Answer from the drawing. Dimensions are ordinates in mm from the lowest x, y and z of the part. A direction names the side the tool comes from. Coordinates: 2 decimals unless noted, no trailing zeros. Order: outer loops, then holes, each group sorted by start corner. A loop starts at its lowest first (then second) coordinate and runs counter-clockwise, first axis right, second up. Notation, with made-up numbers: (18.25, -28.75) -> (38.25, -28.75) arc R10 cw to (38.25, -11.75) -> close; hole circle Ø10 at (48, 78). An arc over 180 degrees is marked (long way). Answer in a Markdown table with one row per item.
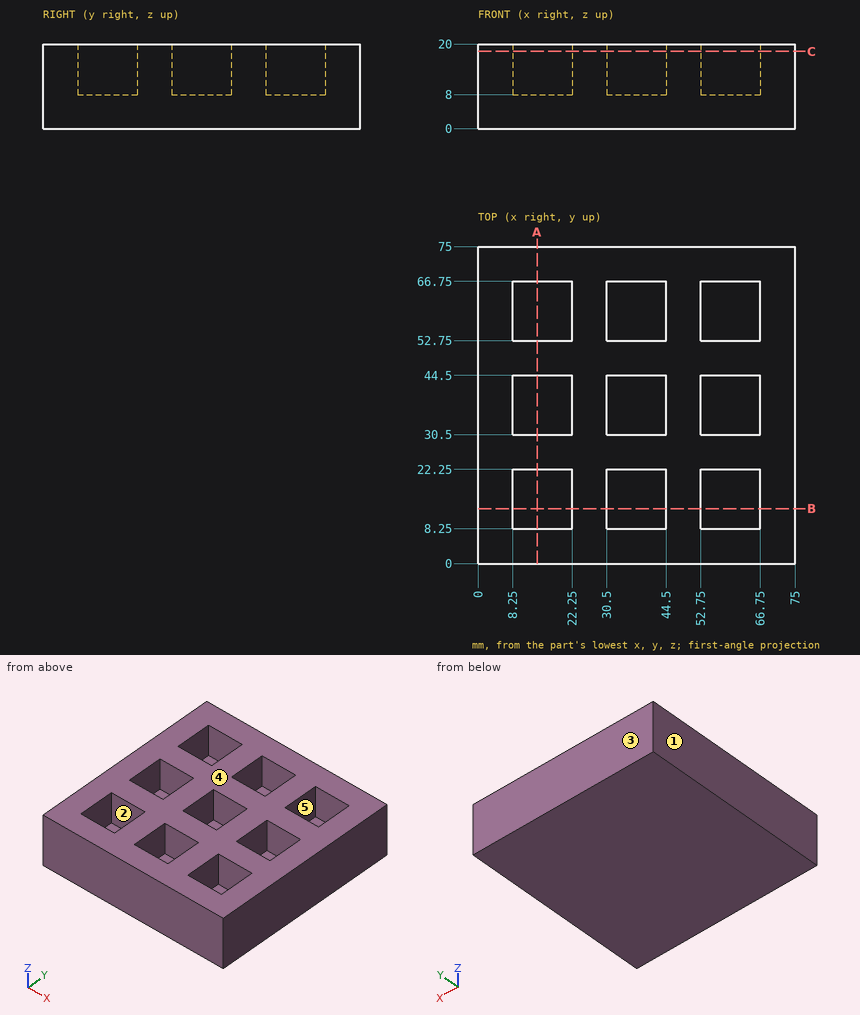
(1) Find the intervals of material crossed by line 1 along Y through (x, z) = (32, 9.75); line 2 along Z through (x, y) = (44, 31), in increasing order. Write a range as from..to.
Check values:
| item | result |
|---|---|
| line 1 | 0..8.25, 22.25..30.5, 44.5..52.75, 66.75..75 |
| line 2 | 0..8 |
(2) A cutting plane is placed at C-C, the plane z = 18.25. Count the separate pieces of the cut face and the enclosed holes in it, then the cut area to 3 significant figures.
Check values:
| item | result |
|---|---|
| separate pieces | 1 |
| enclosed holes | 9 |
| area | 3,860 mm² |
(3) A cutting plane is placed at A-A, the plane x = 14. Determine the outline of the cut face in (y, z).
Check values:
| item | result |
|---|---|
| outline | (0, 0) -> (75, 0) -> (75, 20) -> (66.75, 20) -> (66.75, 8) -> (52.75, 8) -> (52.75, 20) -> (44.5, 20) -> (44.5, 8) -> (30.5, 8) -> (30.5, 20) -> (22.25, 20) -> (22.25, 8) -> (8.25, 8) -> (8.25, 20) -> (0, 20) -> close |
(4) For a pull along X with two mould halves and no side action, classify the marked faces 1, 2 and 3 as released by +X, released by -X, zero draft, split by the parting line, or undercut.
Check values:
| item | result |
|---|---|
| face 1 | released by -X |
| face 2 | undercut |
| face 3 | zero draft |
(5) A flat-ended cylindrical pin translates along its axis: pin 1 (4 mm diameter, centred on x = 15.5, y = 15, fed in from +Z). Find the tip coordinate at first contact, or state that the pin passes through.
Check values:
| item | result |
|---|---|
| pin 1 | z = 8 |
(6) Which of the six approach directions +Z, -Z, +X, -X, +Y, -Y give full straight-line access (tool end or side, diameter ignored) to the marked faces 4 and 5?
Check values:
| item | result |
|---|---|
| face 4 | +Z, +X, -X, +Y, -Y |
| face 5 | +Z |
